Build history of the part. All positions in model axes, mm. Face numbers are marked on the shaded views. A direction names the side the tool comes from. Round coordinates to 2 decimals unless told otherwise and drop trailing zeros. Write each loop counter-clockwise with the first axis right and the second up, starting at its lowest first coordinate (ties: lowest second). Pieces come first, ordered by that corner, then holes. Notation, with made-up numbers: M 63.25,64 L 68.25,64 A22 cw 68.25,80 Z; hole C -37.75,-3.5 d8. An arc over 180 degrees is marked long. Use a Markdown table: item, result.
from build123d import *

# Parameters (mm, degrees)
F0_W     = 38.1
F0_H     = 5
F1_DEPTH = 30
F2_R     = 3.175
F3_DEPTH = 25.4


with BuildPart() as f1:
    # F0 (on Top) → F1 (new body)
    with BuildSketch(Plane.XY):
        Polygon((-2.5, -34.925), (2.5, -34.925), (2.5, -29.925), (2.5, 34.925), (-2.5, 34.925), align=None)
        with Locations((21.55, -32.425)):
            Rectangle(F0_W, F0_H)
    extrude(amount=F1_DEPTH)

    # F2 (on face) → F3 (cut)
    with BuildSketch(Plane.YZ.offset(2.5)):
        with Locations((-22.4828, 15)):
            Circle(F2_R)
        with Locations((2.5172, 15)):
            Circle(F2_R)
        with Locations((27.5172, 15)):
            Circle(F2_R)
    extrude(amount=-F3_DEPTH, mode=Mode.SUBTRACT)


solid = f1.part
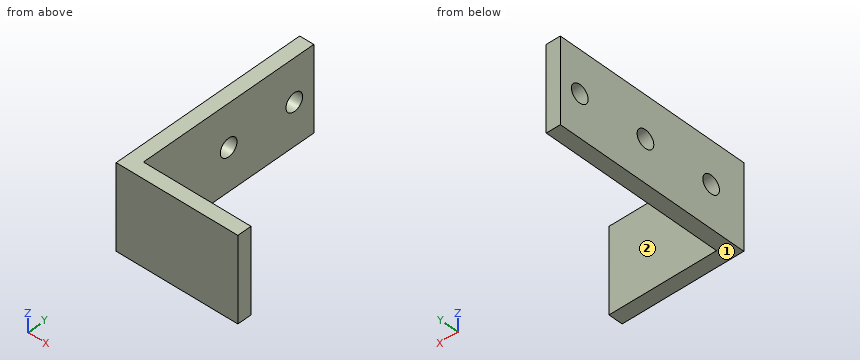
Q1. Which spindle directions (+Z, -Z, +X, -X, +Y, -Y) get a long thin tool onto all of the face, cutting with end or side? Do the marked faces 1 and 2. Say none if no direction does.
Response values:
| item | result |
|---|---|
| face 1 | -Z, +X, -X, +Y, -Y |
| face 2 | +Z, -Z, +X, +Y |
Q2. Cut at C-C on y = -14. Give the cut face in (x, z).
Response values:
| item | result |
|---|---|
| outline | M -2.5,0 L 2.5,0 L 2.5,30 L -2.5,30 Z |
Q3. Cut at B-B on z = 22.25. Give the cut face in (x, y) (3 decimals).
Response values:
| item | result |
|---|---|
| outline | M -2.5,-34.925 L 40.6,-34.925 L 40.6,-29.925 L 2.5,-29.925 L 2.5,34.925 L -2.5,34.925 Z |
Q4. Cut at A-A on z = 16.25. Give the cut face in (x, y) (3 decimals).
Response values:
| item | result |
|---|---|
| outline | M -2.5,-34.925 L 40.6,-34.925 L 40.6,-29.925 L 2.5,-29.925 L 2.5,-25.401 L -2.5,-25.401 Z; M -2.5,-19.564 L 2.5,-19.564 L 2.5,-0.401 L -2.5,-0.401 Z; M -2.5,5.436 L 2.5,5.436 L 2.5,24.599 L -2.5,24.599 Z; M -2.5,30.436 L 2.5,30.436 L 2.5,34.925 L -2.5,34.925 Z |
Q5. Cut at D-D on x = 6.5. Give the cut face in (y, z) (3 decimals), and give its area (3 significant figures).
Response values:
| item | result |
|---|---|
| outline | M -34.925,0 L -29.925,0 L -29.925,30 L -34.925,30 Z |
| area | 150 mm2 |
Q6. Drill centre lines: L1, parallel to Y at x = 27.5, z = 9.5 (3 decimals); L2, parallel to X at y = 31.5, z = 9.5; L3, parallel to Z at x = 0, y = 25. Where is each one in solid material? Low to high.
Response values:
| item | result |
|---|---|
| L1 | y = -34.925 to -29.925 |
| L2 | x = -2.5 to 2.5 |
| L3 | z = 0 to 13.06, 16.94 to 30 |
Q7. Drop flat-ended pins along their axis: P1, Ø7.5, axis at y = 2.52, z = 15, coming from the +X side; P2, Ø1, axis at x = 6, z = 7.5, coming from the +Y side (3 decimals). Give the stop position or say it passes through.
Response values:
| item | result |
|---|---|
| P1 | stops at x = 2.5 |
| P2 | stops at y = -29.925 |
